```python
from build123d import *

# Parameters (mm, degrees)
CUT_EXTRUDE1_DEPTH = 10


with BuildPart() as part:
    # Sketch1 → Loft4 section 0
    with BuildSketch(Plane(origin=(0, 0, 0), x_dir=(0, 0, -1), z_dir=(1, 0, 0))):
        Polygon((-205, 500), (195, 500), (195, 490), (0, 490), (0, -490), (195, -490), (195, -500), (-205, -500), (-205, -490), (-10, -490), (-10, 490), (-205, 490), align=None)
    # Sketch4 → Loft4 section 1
    with BuildSketch(Plane(origin=(1000, 0, -1000), x_dir=(0, 0, 1), z_dir=(-1, 0, 0))):
        Polygon((805, 400), (1205, 400), (1205, 390), (1010, 390), (1010, -390), (1205, -390), (1205, -400), (805, -400), (805, -390), (1000, -390), (1000, 390), (805, 390), align=None)
    loft()

    # Sketch6 → Cut-Extrude1 (cut)
    with BuildSketch(Plane.XY.offset(10)):
        with BuildLine():
            Line((215.970223141, -317.654843369), (795.970223141, -259.654843369))
            ThreePointArc((795.970223141, -259.654843369), (834.487152013, -240.212931202), (850, -199.952611956))
            Line((850, -199.952611956), (850, 199.952611956))
            ThreePointArc((850, 199.952611956), (834.487152013, 240.212931202), (795.970223141, 259.654843369))
            Line((795.970223141, 259.654843369), (215.970223141, 317.654843369))
            ThreePointArc((215.970223141, 317.654843369), (169.739680754, 302.43976397), (150, 257.952611956))
            Line((150, 257.952611956), (150, -257.952611956))
            ThreePointArc((150, -257.952611956), (169.739680754, -302.43976397), (215.970223141, -317.654843369))
        make_face()
    extrude(amount=-CUT_EXTRUDE1_DEPTH, mode=Mode.SUBTRACT)


solid = part.part
```
Input: part model. Units: mm. Frame: model coordinates. A direction names the side the tool comes from. Round coordinates to 2 decimals unless told otherwise and drop trailing zeros. Loops run counter-clockwise (first coordinate to the right, second up) from the corner with the lowest first, then second, coordinate; pieces in that order, holes last. Notation, with made-up numbers: (9, 42) - (45, 42) arc R32 ccw to (45, 75) - close; hole circle Ø5 at (32, 60.5). An arc over 180 degrees is marked (long way). One line per item, written item: value. Start each with the question number.
(1) Contact query for flat-ended pins moving along their axis: P1, Ø8, axis at y = -0.5, z = 6, coming from the -X side; P2, Ø6, axis at x = 812.5, z = -63, coming from the -Y side; P3, Ø12, axis at x = 132, z = 158.5, coming from the -Y side; P4, Ø8, axis at x = 267.5, z = -46.5, coming from the -Y side. Output: stop coordinate, or through.
(2) Section A-A, the plane z = 28. Return loops of the section in (x, y), plus the area to 3 significant figures.
(3) Draft query along Y for faces 5 (the flat face through (507, 449.3, 7.8)), 6 (the flat face through (507, -439.3, -96.1)), 7 (the flat face through (0, 3, 4)). Return one class per face: +Y half, -Y half, draft (parallel to the pull), parting line (faces both ways), or undercut.
(4) Access query for faces 1 (the flat face through (507, -449.3, 2.2)), 2 (the flat face through (507, 439.3, 106.1)), 3 (the cylindrical face through (834.9, 239.75, 5.07)), 4 (the flat face through (507, 439.3, -98.9)). Directions: +Z, -Z, +X, -X, +Y, -Y. A direction counts if a zero-diameter tool reaches every point of the face in a straight line with its end or side. Return the directions, or none.
(5) Ray query, line 1 (Z direction, x = 798, y = -268); line 2 (Y direction, x = 354.5, z = 88); line 3 (Y direction, x = 384.5, z = -111). Return the intervals inside material, ascending. Write a range as [from, to].
Results below:
1. P1: x = 0
1. P2: y = -419.05
1. P3: y = -487.4
1. P4: y = -473.65
2. outline: (0, -500) - (1000, -400) - (1000, -390) - (0, -490) - close; (0, 490) - (1000, 390) - (1000, 400) - (0, 500) - close
2. area: 20,000 mm^2
3. face 5: +Y half
3. face 6: undercut
3. face 7: draft
4. face 1: +Z, -Z, +X, -Y
4. face 2: +Z, -X
4. face 3: +Z, -Z
4. face 4: -Z, -X
5. line 1: [0, 10]
5. line 2: [-464.55, -454.55], [454.55, 464.55]
5. line 3: [-461.55, -451.55], [451.55, 461.55]
